Geometry check sheet. Reference: the model listing, model coordinates, mm. A direction names the side the tool comes from. Coordinates: 2 decimals unless noted, no trailing zeros. Write each loop counter-clockwise with the first axis right and the second up, starting at its lowest first coordinate (ties: lowest second). Pieces come first, ordered by that corner, then holes. Notation, with made-up numbers: M 39,-1 L 51,-1 A32 cw 51,28 Z; hole C 86.5,78 d7. An arc over 180 degrees is marked long. Put each result on its own line as item: value. Start each with the question number.
1) Set-up check for faces 1 (the cylindrical face through (-20.04, 0.95, 3.03)), 2 (the conical face through (-13.92, 2.67, 8.48)), 3 (the cylindrical face through (-59.5, 5.55, 9.7)), 4 (the cylindrical face through (-59.5, -5.55, -9.7)): record each of +Z, -Z, +X, -X, +Y, -Y from which the full face is reachable in a straight line by a thin tool's end or side.
2) Scan lines: line 1 along Y through (x, z) = (-26, 0) (3 decimals); line 2 along Z through (x, y) = (-15, 2.5); line 3 along Y through (x, z) = (-20.5, 1.5). Record each from-to range of solid material in increasing order.
3) Gauge pin test, flat ends, axial feed: pin 1 (1 mm diameter, centred on x = -55, y = 10, fed in from +Z); pin 2 (3 mm diameter, centred on y = 1, z = -1, fed in from +X); pin 3 (6 mm diameter, centred on y = 4, z = -8, fed in from -X). Record the tip position at first contact, or that the pin passes through.
4) Cross-section at B-B on y = 0. Record the cut outline in (x, z) (3 decimals).
5) Cross-section at A-A on x = -58.5. Record the cut outline in (y, z), plus the area to 3 significant figures.
6) Cross-section at C-C on x = -18.5. Record the cut outline in (y, z) (3 decimals).
7) Mould release check, pull along X, two halves, no side actions. Record for faces 5 (the cylindrical face through (-32.171, 7.075, -0.457)), 6 (the cylindrical face through (-3.22, -12.4, -2.75)), 7 (the flat face through (-40.64, 0, 0)): released by +X, released by -X, zero draft, split by the parting line, or undercut.
from build123d import *

# Parameters (mm, degrees)
F4_START = -7.62
F4_DEPTH = 93.981
F5_R     = 1.1938
F6_DEPTH = 12.7


with BuildPart() as f1:
    # F0 (on Front) → F1 (revolve)
    with BuildSketch(Plane.XZ):
        with BuildLine():
            Line((-40.64, 3.175), (0, 3.175))
            Line((0, 3.175), (0, 12.7))
            Line((0, 12.7), (-6.35, 12.7))
            Line((-6.35, 12.7), (-6.35, 9.7636567324))
            ThreePointArc((-6.35, 9.7636567324), (-7.4331158517, 7.6830105399), (-9.758731164, 7.3768374756))
            Line((-9.758731164, 7.3768374756), (-24.384, 12.7))
            Line((-24.384, 12.7), (-99.4210244843, 12.7))
            ThreePointArc((-99.4210244843, 12.7), (-101.0513051228, 6.4427853895), (-101.6, 0))
            Line((-101.6, 0), (-40.64, 0))
            Line((-40.64, 0), (-40.64, 3.175))
        make_face()
    revolve(axis=Axis((-71.12, 0, 0), (-1, 0, 0)))

    # F2 (on Right) → F4 (cut)
    with BuildSketch(Plane.YZ.offset(F4_START)):
        with BuildLine():
            ThreePointArc((-3.175, 13.8581385114), (-3.2583413998, 14.751147695), (-3.5054871123, 15.6133136811))
            ThreePointArc((-3.5054871123, 15.6133136811), (-8.001, 13.8581385114), (-11.768782729, 10.8424977325))
            ThreePointArc((-11.768782729, 10.8424977325), (-6.4030393387, 9.3043710903), (-3.175, 13.8581385114))
        make_face()
        with BuildLine():
            ThreePointArc((3.5054871123, 15.6133136811), (5.588, 9.6786999127), (11.768782729, 10.8424977325))
            ThreePointArc((11.768782729, 10.8424977325), (8.001, 13.8581385114), (3.5054871123, 15.6133136811))
        make_face()
        with BuildLine():
            ThreePointArc((15.2742698413, -4.7708159487), (15.8190213035, -2.413), (16.002, 0))
            ThreePointArc((16.002, 0), (15.8190213035, 2.413), (15.2742698413, 4.7708159487))
            ThreePointArc((15.2742698413, 4.7708159487), (11.176, 0), (15.2742698413, -4.7708159487))
        make_face()
        with BuildLine():
            ThreePointArc((3.5054871123, -15.6133136811), (8.001, -13.8581385114), (11.768782729, -10.8424977325))
            ThreePointArc((11.768782729, -10.8424977325), (5.588, -9.6786999127), (3.5054871123, -15.6133136811))
        make_face()
        with BuildLine():
            ThreePointArc((-11.768782729, -10.8424977325), (-8.001, -13.8581385114), (-3.5054871123, -15.6133136811))
            ThreePointArc((-3.5054871123, -15.6133136811), (-3.2583413998, -14.751147695), (-3.175, -13.8581385114))
            ThreePointArc((-3.175, -13.8581385114), (-6.4030393387, -9.3043710903), (-11.768782729, -10.8424977325))
        make_face()
        with BuildLine():
            ThreePointArc((-11.176, 0), (-12.3412417626, 3.1446979389), (-15.2742698413, 4.7708159487))
            ThreePointArc((-15.2742698413, 4.7708159487), (-16.002, 0), (-15.2742698413, -4.7708159487))
            ThreePointArc((-15.2742698413, -4.7708159487), (-12.3412417626, -3.1446979389), (-11.176, 0))
        make_face()
    extrude(amount=-F4_DEPTH, mode=Mode.SUBTRACT)

    # F5 (on Front) → F6 (cut, symmetric)
    with BuildSketch(Plane.XZ):
        with Locations((-33.274, 0)):
            Circle(F5_R)
    extrude(amount=F6_DEPTH, both=True, mode=Mode.SUBTRACT)


solid = f1.part
Answer key:
1. face 1: +X
1. face 2: none
1. face 3: +Z, -X
1. face 4: -Z, -X
2. line 1: y = -11.176 to -3.175, 3.175 to 11.176
2. line 2: z = -8.94 to -1.96, 1.96 to 8.94
2. line 3: y = -11.19 to -2.8, 2.8 to 11.19
3. pin 1: stops at z = 8.43
3. pin 2: stops at x = -40.64
3. pin 3: stops at x = -101.13
4. outline: M -99.421,-12.7 L -24.384,-12.7 L -9.759,-7.377 A2.54 cw -6.35,-9.764 L -6.35,-12.7 L 0,-12.7 L 0,-3.175 L -40.64,-3.175 L -40.64,3.175 L 0,3.175 L 0,12.7 L -6.35,12.7 L -6.35,9.764 A2.54 cw -9.759,7.377 L -24.384,12.7 L -99.421,12.7 A38.1 ccw Z
5. outline: M -12.31,-3.11 A12.7 ccw -8.85,-9.11 A4.83 cw -3.46,-12.22 A12.7 ccw 3.46,-12.22 A4.83 cw 8.85,-9.11 A12.7 ccw 12.31,-3.11 A4.83 cw 12.31,3.11 A12.7 ccw 8.85,9.11 A4.83 cw 3.46,12.22 A12.7 ccw -3.46,12.22 A4.83 cw -8.85,9.11 A12.7 ccw -12.31,3.11 A4.83 cw Z
5. area: 468 mm²
6. outline: C 0,0 d21.117; hole C 0,0 d6.35
7. face 5: undercut
7. face 6: zero draft
7. face 7: released by +X
